```python
from build123d import *

# Parameters (mm, degrees)
SKETCH1_R         = 4.0005
EXTRUDE1_DEPTH    = 2.921
FILLET1_R         = 1.524
SKETCH2_R         = 2.032
EXTRUDE2_DEPTH    = 8.89
SKETCH3_W         = 4.91456988
SKETCH3_H         = 0.615801824
EXTRUDE3_DEPTH    = 1.016
CIRPATTERN1_COUNT = 2
CIRPATTERN1_ANGLE = 90


with BuildPart() as part:
    # Sketch1 → Extrude1 (new body)
    with BuildSketch(Plane.XY):
        Circle(SKETCH1_R)
    extrude(amount=EXTRUDE1_DEPTH)

    # Fillet1
    fillet1_edges = [part.edges().sort_by_distance(p)[0] for p in [
        (-4.0005, 0, 0),
    ]]
    fillet(fillet1_edges, radius=FILLET1_R)

    # Sketch2 → Extrude2 (add)
    with BuildSketch(Plane.XY.offset(2.921)):
        Circle(SKETCH2_R)
    extrude(amount=EXTRUDE2_DEPTH)

    # Sketch3 → Extrude3 (cut)
    with BuildSketch(Plane(origin=(0, 0, 0), x_dir=(-1, 0, 0), z_dir=(0, 0, -1))):
        Rectangle(SKETCH3_W, SKETCH3_H)
    extrude3 = extrude(amount=-EXTRUDE3_DEPTH, mode=Mode.SUBTRACT)

    # CirPattern1: Extrude3 ×2 about axis
    cirpattern1_axis = Axis((0, 0, 0), (0, 0, -1))
    for i in range(1, CIRPATTERN1_COUNT):
        add(extrude3.rotate(cirpattern1_axis, i * CIRPATTERN1_ANGLE / (CIRPATTERN1_COUNT - 1)), mode=Mode.SUBTRACT)


solid = part.part
```
Geometry: final body of the model. Coordinates: model frame, mm. A direction names the side the tool comes from. Coordinates: 2 decimals unless noted, no trailing zeros. Order: outer loops, then holes, each group sorted by start corner. A loop starts at its lowest first (then second) coordinate and runs counter-clockwise, first axis right, second up. Notation, with made-up numbers: (52.5, 19.25) -> (63.5, 19.25) arc R18 ccw to (63.5, 36.25) -> close; hole circle Ø11 at (55.25, 62.5). An arc over 180 degrees is marked (long way). Write each question's results on one line, items separated by ' | '. Start each with the question number.
1) Material intervals for line 1 along Z through (x, y) = (-1.25, -1.75); line 2 along X through (y, z) = (-3, 1); line 3 along X through (y, z) = (-0.5, 9.25), sorted ascending.
2) First-contact query: pin 1 (1.1 mm diameter, centred on x = -1, z = 0.5, fed in from +Y); pin 2 (1.1 mm diameter, centred on y = 1.5, z = 0.5, fed in from -X); pin 3 (2 mm diameter, centred on y = -2, z = 1.5, fed in from -X); pin 4 (4 mm diameter, centred on x = 1, z = 3, fed in from -Y). Flat tips, straight axial feed; report the tip coordinate or a pass-through.
3) Cut plane C-C, the plane z = 4.75. Output: boundary loops of the cut face in (x, y).
4) Set-up query: faces 4 (the flat face through (1.4, 0.308, 0.5)), 5 (the cylindrical face through (-0.44, -1.984, 7.304)), 6 (the flat face through (-1, 1, 0)). Return all of +Z, -Z, +X, -X, +Y, -Y with unobstructed straight access to the full face (end or side cutting, diameter ignored); none if empty.
5) Mould query, pull axis Y, two halves, no side actions, for faces 1 (the flat face through (-0.308, -1.4, 0.5)), 2 (the flat face through (0, 0, 11.811)), 3 (the cylindrical face through (-0.9, -3.9, 2.2)). Classes: released by +Y, released by -Y, zero draft, split by the parting line, or undercut.
Checks:
1) line 1: 0 to 2.92 | line 2: -2.5 to 2.5 | line 3: -1.97 to 1.97
2) pin 1: y = 3.83 | pin 2: x = -3.7 | pin 3: x = -3.87 | pin 4: y = -4
3) outline: circle Ø4.06 at (0, 0)
4) face 4: -Z | face 5: +Z | face 6: -Z, +X, -X, +Y, -Y
5) face 1: undercut | face 2: zero draft | face 3: split by the parting line
